Part model, mm, in its own coordinate system. A direction names the side the tool comes from. Round coordinates to 2 decimals unless told otherwise and drop trailing zeros. Order: outer loops, then holes, each group sorted by start corner. A loop starts at its lowest first (then second) coordinate and runs counter-clockwise, first axis right, second up. Notation, with made-up numbers: (31.5, 34) -> (46.5, 34) arc R21 cw to (46.5, 42) -> close; hole circle Ø2 at (68, 59.5). An arc over 180 degrees is marked (long way). Use CSV: the item, a comma, the result in double quotes.
```python
from build123d import *

# Parameters (mm, degrees)
F1_DEPTH = 5.08
F0_R     = 5.442905
F2_DEPTH = 3.81
F0_R_2   = 1.5875
F3_DEPTH = 3.175


with BuildPart() as f1:
    # F0 (on Top) → F1 (new body)
    with BuildSketch(Plane.XY):
        with BuildLine():
            Line((-21.217541, 1.695553), (-21.167484, 1.695553))
            Line((-21.167484, 1.695553), (-6.632199, 1.695553))
            ThreePointArc((-6.632199, 1.695553), (0, 6.845507), (6.632199, 1.695553))
            Line((6.632199, 1.695553), (21.167484, 1.695553))
            Line((21.167484, 1.695553), (21.217541, 1.695553))
            ThreePointArc((21.217541, 1.695553), (0, 21.285181), (-21.217541, 1.695553))
        make_face()
        with BuildLine():
            Line((-6.648738, -1.629494), (-21.172672, -1.629494))
            Line((-21.172672, -1.629494), (-21.222716, -1.629494))
            ThreePointArc((-21.222716, -1.629494), (0, -21.285181), (21.222716, -1.629494))
            Line((21.222716, -1.629494), (21.172672, -1.629494))
            Line((21.172672, -1.629494), (6.648738, -1.629494))
            ThreePointArc((6.648738, -1.629494), (0, -6.845507), (-6.648738, -1.629494))
        make_face()
    extrude(amount=F1_DEPTH)

    # F0 (on Top) → F2 (join)
    with BuildSketch(Plane.XY):
        with BuildLine():
            ThreePointArc((22.80185, -1.629494), (22.845458, -0.815266), (22.86, 0))
            ThreePointArc((22.86, 0), (22.844253, 0.848361), (22.797033, 1.695553))
            ThreePointArc((22.797033, 1.695553), (17.318605, 14.921311), (5.048545, 22.295556))
            ThreePointArc((5.048545, 22.295556), (0, 22.86), (-5.048545, 22.295556))
            ThreePointArc((-5.048545, 22.295556), (-17.860422, 14.268319), (-22.86, 0))
            ThreePointArc((-22.86, 0), (-1.23935, -22.82638), (22.725618, -2.475054))
            Line((22.725618, -2.475054), (22.725618, -1.629494))
            Line((22.725618, -1.629494), (22.80185, -1.629494))
        make_face()
        with BuildLine():
            Line((-21.222716, -1.629494), (-21.172672, -1.629494))
            Line((-21.172672, -1.629494), (-6.648738, -1.629494))
            ThreePointArc((-6.648738, -1.629494), (0, -6.845507), (6.648738, -1.629494))
            Line((6.648738, -1.629494), (21.172672, -1.629494))
            Line((21.172672, -1.629494), (21.222716, -1.629494))
            ThreePointArc((21.222716, -1.629494), (0, -21.285181), (-21.222716, -1.629494))
        make_face(mode=Mode.SUBTRACT)
        Circle(F0_R, mode=Mode.SUBTRACT)
        with BuildLine():
            Line((-6.632199, 1.695553), (-21.167484, 1.695553))
            Line((-21.167484, 1.695553), (-21.217541, 1.695553))
            ThreePointArc((-21.217541, 1.695553), (0, 21.285181), (21.217541, 1.695553))
            Line((21.217541, 1.695553), (21.167484, 1.695553))
            Line((21.167484, 1.695553), (6.632199, 1.695553))
            ThreePointArc((6.632199, 1.695553), (0, 6.845507), (-6.632199, 1.695553))
        make_face(mode=Mode.SUBTRACT)
    extrude(amount=F2_DEPTH)

    # F0 (on Top) → F3 (join)
    with BuildSketch(Plane.XY):
        with BuildLine():
            ThreePointArc((-5.048545, 22.295556), (0, 22.86), (5.048545, 22.295556))
            ThreePointArc((5.048545, 22.295556), (0, 27.94), (-5.048545, 22.295556))
        make_face()
        with Locations((0, 25.717106)):
            Circle(F0_R_2, mode=Mode.SUBTRACT)
    extrude(amount=F3_DEPTH)


solid = f1.part
```
(1) Drop flat-ended pins along their axis: P1, Ø1, axis at y = 11.5, z = 2, coming from the -X side; P2, Ø2, axis at x = -3, z = 2.5, coming from the +Y side; P3, Ø1, axis at x = -16.5, z = 4.5, coming from the -Y side; P4, Ø1.5, axis at x = -15, y = -3, coming from the -Z side. Give the stop position or say it passes through.
Reply:
P1,"x = -20.04"
P2,"y = 27.53"
P3,"y = -14.04"
P4,"z = 0"
(2) Cut at A-A, the plane x = 0. Give the cut face in (y, z) (1 decimal).
Reply:
outline,"(-22.9, 0) -> (-5.4, 0) -> (-5.4, 3.8) -> (-6.8, 3.8) -> (-6.8, 5.1) -> (-21.3, 5.1) -> (-21.3, 3.8) -> (-22.9, 3.8) -> close; (5.4, 0) -> (24.1, 0) -> (24.1, 3.2) -> (22.9, 3.2) -> (22.9, 3.8) -> (21.3, 3.8) -> (21.3, 5.1) -> (6.8, 5.1) -> (6.8, 3.8) -> (5.4, 3.8) -> close; (27.3, 0) -> (27.9, 0) -> (27.9, 3.2) -> (27.3, 3.2) -> close"
(3) Which spindle directions (+Z, -Z, +X, -X, +Y, -Y) get a long thin tool onto all of the face, cutting with end or side? Do faces 1 (the face through (14, -1.629, 4)), 2 (the face through (5, 3, 0)), 3 (the face through (0.44, 21.28, 4.44)), 4 (the face through (0.127, -6.844, 4.436)), 5 (the face through (-1.18, -5.313, 1.878)). Say none if no direction does.
Reply:
face 1,"+Z, +X, -X"
face 2,"-Z, +X, -X, +Y, -Y"
face 3,"+Z, +Y"
face 4,"+Z"
face 5,"+Z, -Z"
(4) Pull direction Y, two halves, no side cores. Call faces 6 (the face through (-0.45, -21.28, 4.44)), 7 (the face through (0, -11, 5.08)), 8 (the face through (-5, -3, 3.81)): released by +Y, released by -Y, zero draft, split by the parting line, or undercut.
Reply:
face 6,"released by -Y"
face 7,"zero draft"
face 8,"undercut"
(5) Cut at C-C, the plane y = -15. Give the cut face in (x, z).
Reply:
outline,"(-17.25, 0) -> (17.25, 0) -> (17.25, 3.81) -> (15.1, 3.81) -> (15.1, 5.08) -> (-15.1, 5.08) -> (-15.1, 3.81) -> (-17.25, 3.81) -> close"
(6) Cut at D-D, the plane x = -8. Give the cut face in (y, z), then the cut area to 3 significant figures.
Reply:
outline,"(-21.41, 0) -> (21.41, 0) -> (21.41, 3.81) -> (19.72, 3.81) -> (19.72, 5.08) -> (1.7, 5.08) -> (1.7, 3.81) -> (-1.63, 3.81) -> (-1.63, 5.08) -> (-19.72, 5.08) -> (-19.72, 3.81) -> (-21.41, 3.81) -> close"
area,"209 mm2"
(7) Probe probe 1 along Y at (x, z) = (0, 1.6); probe 2 along Y at (x, z) = (0.5, 1.2); probe 3 along Y at (x, z) = (1, 3.75). List the from-to ranges inside material, lowest first. Write a range as [from, to].
Reply:
probe 1,"[-22.86, -5.44], [5.44, 24.13], [27.3, 27.94]"
probe 2,"[-22.85, -5.42], [5.42, 24.21], [27.22, 27.92]"
probe 3,"[-22.84, -5.35], [5.35, 22.84]"
(8) Cut at B-B, the plane z = 1. State how many separate pieces and enclosed holes the cut face has, then the cut area to 3 significant figures.
Reply:
separate pieces,"1"
enclosed holes,"2"
area,"1,580 mm2"
